Could you check a few things on this model? Use its own coordinates, in mm. A direction names the side the tool comes from. Give positions to 0.01 mm unless a question says otherwise; leave off trailing zeros. Order: outer loops, then holes, each group sorted by start corner. A loop starts at its lowest first (then second) coordinate and runs counter-clockwise, first axis right, second up.
from build123d import *

# Parameters (mm, degrees)
F0_W     = 90
F0_H     = 103
F1_DEPTH = 3
F3_DEPTH = 3


with BuildPart() as f1:
    # F0 (on Top) → F1 (new body)
    with BuildSketch(Plane.XY):
        Rectangle(F0_W, F0_H)
        with BuildLine():
            ThreePointArc((-22.982442, -46.499999), (-27.534895, -43.567646), (-26.747589, -38.210065))
            Line((-26.747589, -38.210065), (-3.765147, -11.907937))
            ThreePointArc((-3.765147, -11.907937), (0, -10.197872), (3.765147, -11.907937))
            Line((3.765147, -11.907937), (26.747588, -38.210065))
            ThreePointArc((26.747588, -38.210065), (27.534895, -43.567646), (22.982441, -46.499999))
            Line((22.982441, -46.499999), (-22.982442, -46.499999))
        make_face(mode=Mode.SUBTRACT)
        with BuildLine():
            ThreePointArc((-40, 24.857684), (-36.757024, 29.538802), (-31.234853, 28.147618))
            Line((-31.234853, 28.147618), (-9.514547, 3.289934))
            ThreePointArc((-9.514547, 3.289934), (-8.279694, 0), (-9.514547, -3.289934))
            Line((-9.514547, -3.289934), (-31.234853, -28.147618))
            ThreePointArc((-31.234853, -28.147618), (-36.757024, -29.538802), (-40, -24.857684))
            Line((-40, -24.857684), (-40, 24.857684))
        make_face(mode=Mode.SUBTRACT)
        with BuildLine():
            Line((9.514547, 3.289934), (31.234853, 28.147618))
            ThreePointArc((31.234853, 28.147618), (36.757024, 29.538802), (40, 24.857684))
            Line((40, 24.857684), (40, -24.857684))
            ThreePointArc((40, -24.857684), (36.757024, -29.538802), (31.234853, -28.147618))
            Line((31.234853, -28.147618), (9.514547, -3.289934))
            ThreePointArc((9.514547, -3.289934), (8.279694, 0), (9.514547, 3.289934))
        make_face(mode=Mode.SUBTRACT)
        with BuildLine():
            ThreePointArc((22.982441, 46.499999), (27.534895, 43.567646), (26.747588, 38.210065))
            Line((26.747588, 38.210065), (3.765147, 11.907937))
            ThreePointArc((3.765147, 11.907937), (0, 10.197872), (-3.765147, 11.907937))
            Line((-3.765147, 11.907937), (-26.747589, 38.210065))
            ThreePointArc((-26.747589, 38.210065), (-27.534895, 43.567646), (-22.982442, 46.499999))
            Line((-22.982442, 46.499999), (22.982441, 46.499999))
        make_face(mode=Mode.SUBTRACT)
    extrude(amount=F1_DEPTH)

    # F2 (on face) → F3 (join, through all)
    with BuildSketch(Plane.XY.offset(3)):
        Polygon((-45, 33.5), (-45, 45.5), (-51, 45.5), (-51, 30.5), (-48, 30.5), (-48, 33.5), align=None)
        Polygon((51, 45.5), (45, 45.5), (45, 33.5), (48, 33.5), (48, 30.5), (51, 30.5), align=None)
        Polygon((51, -29.5), (45, -29.5), (45, -41.5), (48, -41.5), (48, -44.5), (51, -44.5), align=None)
        Polygon((-45, -41.5), (-45, -29.5), (-51, -29.5), (-51, -44.5), (-48, -44.5), (-48, -41.5), align=None)
    extrude(amount=-F3_DEPTH)


solid = f1.part
Item 1: For faces 4 (the flat face through (48, 32, 2)), 5 (the flat face through (-50, -44.5, 2)), 6 (the flat face through (48, -43, 2)), which set-ups out of +Z, -Z, +X, -X, +Y, -Y let a thin tool reach every point of the face, with its end or its side?
Findings:
face 4: +Z, -Z
face 5: +Z, -Z, -X, -Y
face 6: +Z, -Z, -Y
Item 2: Please list where these lines run through material, in increasing order: line 1 along X through (y, z) = (5.5, 2.4); line 2 along X through (y, z) = (7, 2.7); line 3 along Y through (x, z) = (24.5, 1.7).
Findings:
line 1: x = -45 to -40, -11.45 to 11.45, 40 to 45
line 2: x = -45 to -40, -12.76 to 12.76, 40 to 45
line 3: y = -51.5 to -46.26, -35.64 to -20.44, 20.44 to 35.64, 46.26 to 51.5
Item 3: We'd pull the mould along Y, two halves only. Please class faces 1 (the flat face through (45, 48, 1)), 2 (the flat face through (46, -41.5, 2)), 3 (the cylindrical face through (-0.1, -10.2, 1.5)): +Y half, -Y half, draft (parallel to the pull), parting line (faces both ways), or undercut.
Findings:
face 1: draft
face 2: -Y half
face 3: undercut
Item 4: Imagine slicing it at D-D on y = 15. List the corners of the cut face in (x, z) for me, then the cut area to 3 significant figures.
Findings:
outline: (-45, 0) - (-40, 0) - (-40, 3) - (-45, 3) - close; (-19.75, 0) - (-6.47, 0) - (-6.47, 3) - (-19.75, 3) - close; (6.47, 0) - (19.75, 0) - (19.75, 3) - (6.47, 3) - close; (40, 0) - (45, 0) - (45, 3) - (40, 3) - close
area: 110 mm2
Item 5: For pin 1 (1.5 mm diameter, centred on y = 48.5, z = 2, fed in from -X); pin 2 (1.5 mm diameter, centred on x = -48, z = 2, fed in from +Y); pin 3 (0.9 mm diameter, centred on x = -47, z = 2, fed in from -Y), each with a flat end and sliding along its axis, tell me the tip position at first contact or that it passes through.
Findings:
pin 1: stops at x = -45
pin 2: stops at y = 45.5
pin 3: stops at y = -41.5
Item 6: Imagine slicing it at A-A on y = 0. List the corners of the cut face in (x, z) for me.
Findings:
outline: (-45, 0) - (-40, 0) - (-40, 3) - (-45, 3) - close; (-8.28, 0) - (8.28, 0) - (8.28, 3) - (-8.28, 3) - close; (40, 0) - (45, 0) - (45, 3) - (40, 3) - close
Item 7: Imagine slicing it at C-C on x = 12. List the corners of the cut face in (y, z) for me, then the cut area to 3 significant figures.
Findings:
outline: (-51.5, 0) - (-46.5, 0) - (-46.5, 3) - (-51.5, 3) - close; (-21.33, 0) - (-6.13, 0) - (-6.13, 3) - (-21.33, 3) - close; (6.13, 0) - (21.33, 0) - (21.33, 3) - (6.13, 3) - close; (46.5, 0) - (51.5, 0) - (51.5, 3) - (46.5, 3) - close
area: 121 mm2
Item 8: Imagine slicing it at B-B on x = 0. List the corners of the cut face in (y, z) for me.
Findings:
outline: (-51.5, 0) - (-46.5, 0) - (-46.5, 3) - (-51.5, 3) - close; (-10.2, 0) - (10.2, 0) - (10.2, 3) - (-10.2, 3) - close; (46.5, 0) - (51.5, 0) - (51.5, 3) - (46.5, 3) - close
